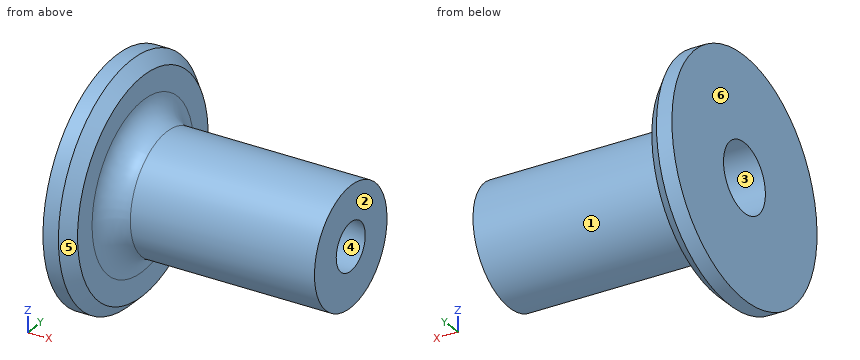
from build123d import *

# Parameters (mm, degrees)
F2_R      = 2
F3_SIZE   = 1
F1_FACE_R = 2.881635
F4_DEPTH  = 25


with BuildPart() as f1:
    # F0 (on Front) → F1 (revolve)
    with BuildSketch(Plane.XZ):
        Polygon((0, 10), (0, 0), (2.3, 0), (2.3, 5), (2.3, 10), align=None)
        Polygon((2.3, 5), (2.3, 0), (14.8, 0), (14.8, 2.881635), (19.8, 2), (19.8, 5), align=None)
    revolve(axis=Axis((11.05, 0, 0), (1, 0, 0)))

    # F2
    f2_edges = [f1.edges().sort_by_distance(p)[0] for p in [
        (2.3, 0, -5),
    ]]
    fillet(f2_edges, radius=F2_R)

    # F3
    f3_edges = [f1.edges().sort_by_distance(p)[0] for p in [
        (2.3, 0, -10),
    ]]
    chamfer(f3_edges, length=F3_SIZE)

    # F1_face (on face) → F4 (cut)
    with BuildSketch(Plane.YZ.offset(14.8)):
        Circle(F1_FACE_R)
    extrude(amount=-F4_DEPTH, mode=Mode.SUBTRACT)


solid = f1.part
Check sheet for the modelled part. Datum: model origin and axes. Units: mm. Face numbers are marked on the shaded views. A direction names the side the tool comes from. Round coordinates to 2 decimals unless told otherwise and drop trailing zeros. Loops run counter-clockwise (first coordinate to the right, second up) from the corner with the lowest first, then second, coordinate; pieces in that order, holes last. Notation, with made-up numbers: M 8.25,52.25 L 43.25,52.25 A23 ccw 43.25,60.25 Z; hole C 35,-34.75 d5. An arc over 180 degrees is marked long. One line per question, with ' | ' between items. Start each with the question number.
Item 1: Gauge pin test, flat ends, axial feed: pin 1 Ø1.5 at (x, y) = (11, 0.5) entering from +Z; pin 2 Ø1.5 at (x, y) = (14, 2.5) entering from +Z; pin 3 Ø6 at (x, y) = (12, -5) entering from -Z. Record the tip position at first contact, or that the pin passes through.
Item 2: Set-up check for the marked faces 1, 2 and 3: record each of +Z, -Z, +X, -X, +Y, -Y from which the full face is reachable in a straight line by a thin tool's end or side.
Item 3: Section check D-D (x = 3). Record the boundary of the cut face in (y, z).
Item 4: Section check A-A (z = 0). Record the boundary of the cut face in (x, y).
Item 5: Release check for a two-part mould opening along Z. For the marked faces 4, 5 and 6 record: released by +Z, released by -Z, zero draft, split by the parting line, or undercut.
Item 6: Scan lines: probe 1 along Z at (x, y) = (7.5, 0); probe 2 along X at (y, z) = (0.5, -8.75). Record each from-to range of solid material in increasing order.
Item 7: Section check C-C (x = 10). Record the boundary of the cut face in (y, z).
Worked out:
1) pin 1: z = 5 | pin 2: z = 4.68 | pin 3: z = -4.58
2) face 1: +X | face 2: +Z, -Z, +X, +Y, -Y | face 3: -X
3) outline: C 0,0 d10.96; hole C 0,0 d5.76
4) outline: M 0,-10 L 1.3,-10 L 2.3,-9 L 2.3,-7 A2 cw 4.3,-5 L 19.8,-5 L 19.8,-2 L 14.8,-2.88 L 0,-2.88 Z; M 0,2.88 L 14.8,2.88 L 19.8,2 L 19.8,5 L 4.3,5 A2 cw 2.3,7 L 2.3,9 L 1.3,10 L 0,10 Z
5) face 4: undercut | face 5: split by the parting line | face 6: zero draft
6) probe 1: -5 to -2.88, 2.88 to 5 | probe 2: 0 to 2.3
7) outline: C 0,0 d10; hole C 0,0 d5.76
